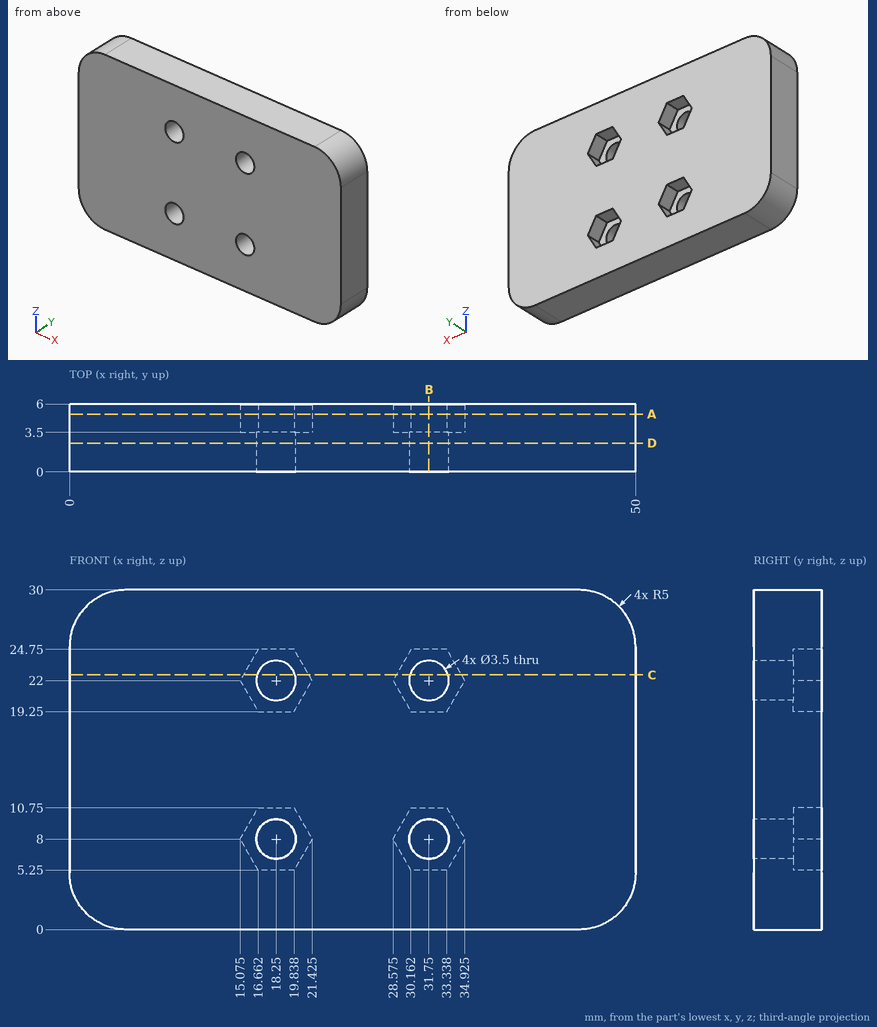
The figure shows three views and two pictorial views of one solid part (mm, origin at its lowest corner). Answer the questions. Round coordinates to 2 decimals unless told otherwise and drop trailing zeros. Write each loop counter-clockwise with the first axis right and the second up, starting at its lowest first coordinate (ties: lowest second). Pieces come first, ordered by that corner, then holes. Notation, with made-up numbers: (68, 79.25) - (87, 79.25) arc R12 ccw to (87, 97.25) - close; hole circle Ø7 at (26, -1.75). An arc over 180 degrees is marked (long way). Answer in a Markdown table with one row per item. Add a question column.
1. A cutting plane is placed at C-C, the plane z = 22.5. Determine the outline of the cut face in (x, y), and give its area (3 significant figures).
2. Find the intervals of material crossed by line 1 along Z through (x, y) = (31.75, 0.85); line 2 along X through (y, z) = (2.3, 8); line 3 along Z through (x, y) = (33, 0.35) (1 decimal), in increasing order. Write a range as from..to.
3. A cutting plane is placed at A-A, the plane y = 5.1. Count the separate pieces of the cut face and the enclosed holes in it, and give its area (3 significant figures).
4. A cutting plane is placed at B-B, the plane x = 31.75. Determine the outline of the cut face in (y, z).
5. A cutting plane is placed at D-D, the plane y = 2.55. Determine the outline of the cut face in (x, z).
6. Given pin 1 (2 mm diameter, centred on x = 31.75, z = 22, fed in from +Y) (3 decimals); pin 2 (5 mm diameter, centred on x = 25, z = 6, fed in from -Y); pin 3 (1.6 mm diameter, centred on x = 19.5, z = 9, fed in from +Y), each flat-ended and moving along its own axis, determine where each tip first touches the part or whether it passes through.
Worked out:
| question | item | result |
|---|---|---|
| 1 | outline | (0, 0) - (16.57, 0) - (16.57, 3.5) - (15.36, 3.5) - (15.36, 6) - (0, 6) - close; (19.93, 0) - (30.07, 0) - (30.07, 3.5) - (28.86, 3.5) - (28.86, 6) - (21.14, 6) - (21.14, 3.5) - (19.93, 3.5) - close; (33.43, 0) - (50, 0) - (50, 6) - (34.64, 6) - (34.64, 3.5) - (33.43, 3.5) - close |
| 1 | area | 248 mm^2 |
| 2 | line 1 | 0..6.25, 9.75..20.25, 23.75..30 |
| 2 | line 2 | 0..16.5, 20..30, 33.5..50 |
| 2 | line 3 | 0..6.8, 9.2..20.8, 23.2..30 |
| 3 | separate pieces | 1 |
| 3 | enclosed holes | 4 |
| 3 | area | 1,370 mm^2 |
| 4 | outline | (0, 0) - (6, 0) - (6, 5.25) - (3.5, 5.25) - (3.5, 6.25) - (0, 6.25) - close; (0, 9.75) - (3.5, 9.75) - (3.5, 10.75) - (6, 10.75) - (6, 19.25) - (3.5, 19.25) - (3.5, 20.25) - (0, 20.25) - close; (0, 23.75) - (3.5, 23.75) - (3.5, 24.75) - (6, 24.75) - (6, 30) - (0, 30) - close |
| 5 | outline | (0, 5) arc R5 ccw to (5, 0) - (45, 0) arc R5 ccw to (50, 5) - (50, 25) arc R5 ccw to (45, 30) - (5, 30) arc R5 ccw to (0, 25) - close; hole circle Ø3.5 at (18.25, 8); hole circle Ø3.5 at (18.25, 22); hole circle Ø3.5 at (31.75, 8); hole circle Ø3.5 at (31.75, 22) |
| 6 | pin 1 | through |
| 6 | pin 2 | y = 0 |
| 6 | pin 3 | y = 3.5 |
